Geometry: final body of the model. Coordinates: model frame, mm. A direction names the side the tool comes from. Give positions to 0.01 mm unless a question says otherwise; leave off trailing zeros. Write each loop counter-clockwise with the first axis right and the second up, starting at its lowest first coordinate (ties: lowest second). Pieces come first, ordered by that corner, then holes. Notation, with made-up numbers: M 74.5,-31 L 108.5,-31 A14 cw 108.5,-18 Z; hole C 43.25,-15 d3. An arc over 180 degrees is marked long. Use a Markdown table: item, result. Add a question column.
(1) Pin query (flat end, axial travel): pin 1 Ø5.5 at (x, z) = (0, -1) entering from -Y; pin 2 Ø2 at (x, y) = (-2, 1) entering from -Z; pin 3 Ø1 at (y, z) = (3, 2.5) entering from -X; pin 4 Ø2 at (x, y) = (3, -3.5) entering from -Z. Return the tip coordinate at first contact, or that it passes through.
(2) Cut plane C-C (x = 0). Output: boundary loops of the cut face in (y, z).
(3) Cut plane A-A (y = -2.25). Output: boundary loops of the cut face in (x, z).
(4) Reachability of faces 1 (the flat face through (-3, -2, -0.35)), 2 (the cylindrical face through (-1.17, 0.99, 5.27)), 3 (the flat face through (3, -2, 0.35)), 4 (the cylindrical face through (-1.08, 5.28, 4.88)) from +Z, -Z, +X, -X, +Y, -Y: full face, straight path, thin tool, end or side. Return the list, or none.
(5) Cut plane D-D (y = 5.5). Output: boundary loops of the cut face in (x, z), plus the area to 3 significant figures.
(6) Cut plane B-B (z = 0). Output: boundary loops of the cut face in (x, y).
(7) Material intervals for L1, parallel to X at y = -1.75, z = -0.25; L2, parallel to Z at x = 2.25, y = -1.25; L3, parallel to Y at x = 2.25, z = 4.5, sorted ascending.
```python
from build123d import *

# Parameters (mm, degrees)
SKETCH2_W                = 2
SKETCH2_H                = 0.7
BOSS_EXTRUDE1_DEPTH      = 5
BOSS_EXTRUDE1_DEPTH_BACK = 5


with BuildPart() as part:
    # Sketch1 → Revolve1 (revolve)
    with BuildSketch(Plane.XY):
        with BuildLine():
            Line((0, 0), (0, 13.65))
            ThreePointArc((0, 13.65), (3.535533906, 12.185533906), (5, 8.65))
            Line((5, 8.65), (5, 2))
            Line((5, 2), (5.4, 2))
            Line((5.4, 2), (5.4, 0))
            Line((5.4, 0), (0, 0))
        make_face()
    revolve(axis=Axis((0, 0, 0), (0, 1, 0)))

    # Sketch2 → Boss-Extrude1 (add, two sides)
    with BuildSketch(Plane.XZ) as boss_extrude1_sk:
        with Locations((2.54, 0)):
            Rectangle(SKETCH2_W, SKETCH2_H)
        with Locations((-2.54, 0)):
            Rectangle(SKETCH2_W, SKETCH2_H)
    extrude(amount=BOSS_EXTRUDE1_DEPTH)
    extrude(boss_extrude1_sk.sketch, amount=-BOSS_EXTRUDE1_DEPTH_BACK)


solid = part.part
```
Answer list:
| question | item | result |
|---|---|---|
| 1 | pin 1 | y = -5 |
| 1 | pin 2 | z = -5.31 |
| 1 | pin 3 | x = -4.58 |
| 1 | pin 4 | z = -0.35 |
| 2 | outline | M 0,-5.4 L 2,-5.4 L 2,-5 L 8.65,-5 A5 ccw 8.65,5 L 2,5 L 2,5.4 L 0,5.4 Z |
| 3 | outline | M -3.54,-0.35 L -1.54,-0.35 L -1.54,0.35 L -3.54,0.35 Z; M 1.54,-0.35 L 3.54,-0.35 L 3.54,0.35 L 1.54,0.35 Z |
| 4 | face 1 | -Z, +X, -X, -Y |
| 4 | face 2 | +Y, -Y |
| 4 | face 3 | +Z, +X, -X, -Y |
| 4 | face 4 | +Y |
| 5 | outline | C 0,0 d10 |
| 5 | area | 78.5 mm² |
| 6 | outline | M -5.4,0 L -3.54,0 L -3.54,-5 L -1.54,-5 L -1.54,0 L 1.54,0 L 1.54,-5 L 3.54,-5 L 3.54,0 L 5.4,0 L 5.4,2 L 5,2 L 5,8.65 A5 ccw -5,8.65 L -5,2 L -5.4,2 Z |
| 7 | L1 | -3.54 to -1.54, 1.54 to 3.54 |
| 7 | L2 | -0.35 to 0.35 |
| 7 | L3 | 0 to 2 |
